Verification items for this drawing (mm, ordinates from the low corner). Coordinates: 2 decimals unless noted, no trailing zeros. Order: outer loops, then holes, each group sorted by start corner. A loop starts at its lowest first (then second) coordinate and runs counter-clockwise, first axis right, second up. Notation, with made-up numbers: (69, 60.25) -> (108, 60.25) arc R6 ccw to (108, 64.25) -> close; hole circle Ø6 at (-7.75, -8.75). An arc over 180 degrees is marked (long way). Answer as CSV lines item,"result". Start each with the question number.
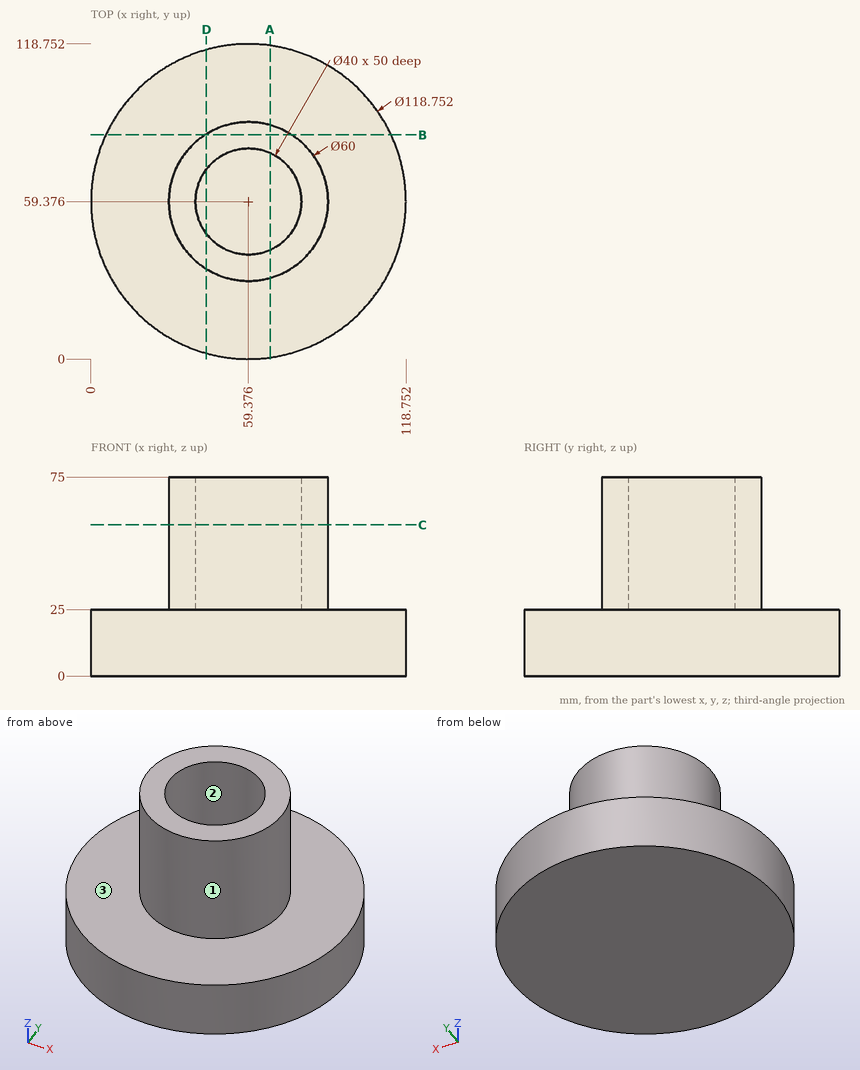
Q1. Sectioned sample at D-D, the plane x = 43.5. Record the cut outline in (y, z), then the cut area to 3 significant figures.
Q2. Go/stop test with flat-tipped pins: pin 1 Ø10 at (x, z) = (65.5, 16) entering from -Y; pin 2 Ø10 at (y, z) = (96.5, 20) entering from +X; pin 3 Ø10 at (x, z) = (85.5, 54.5) entering from -Y (1 decimal). Record where each tip stops, or that it passes through.
Q3. Sectioned sample at B-B, the plane y = 84.5. Record the cut outline in (x, z).
Q4. Sectioned sample at C-C, the plane z = 57. Record the cut outline in (x, y).
Q5. Sectioned sample at A-A, the plane x = 67.5. Record the cut outline in (y, z) (1 decimal), then the cut area to 3 significant figures.
Q6. Thickness scan on L1, parallel to Z at x = 92.5, y = 91; L2, parallel to Y at x = 45, z = 43 (1 decimal); L3, parallel to Y at x = 65, z = 32.5. Record the ranges inside material, lowest first.
Q7. Release check for a two-part mould opening along X. For the marked faces 1, 2 and 3 record: released by +X, released by -X, zero draft, split by the parting line, or undercut.
Geometry results:
1,outline,"(2.16, 0) -> (116.59, 0) -> (116.59, 25) -> (84.83, 25) -> (84.83, 75) -> (71.54, 75) -> (71.54, 25) -> (47.21, 25) -> (47.21, 75) -> (33.92, 75) -> (33.92, 25) -> (2.16, 25) -> close"
1,area,"4,190 mm^2"
2,pin 1,"stops at y = 0.01"
2,pin 2,"stops at x = 109.31"
2,pin 3,"stops at y = 38.1"
3,outline,"(5.58, 0) -> (113.17, 0) -> (113.17, 25) -> (75.77, 25) -> (75.77, 75) -> (42.98, 75) -> (42.98, 25) -> (5.58, 25) -> close"
4,outline,"circle Ø60 at (59.38, 59.38); hole circle Ø40 at (59.38, 59.38)"
5,outline,"(0.6, 0) -> (118.2, 0) -> (118.2, 25) -> (88.3, 25) -> (88.3, 75) -> (77.7, 75) -> (77.7, 25) -> (41.1, 25) -> (41.1, 75) -> (30.5, 75) -> (30.5, 25) -> (0.6, 25) -> close"
5,area,"4,000 mm^2"
6,L1,"z = 0 to 25"
6,L2,"y = 33 to 45.5, 73.3 to 85.7"
6,L3,"y = 29.91 to 40.18, 78.57 to 88.84"
7,face 1,"split by the parting line"
7,face 2,"undercut"
7,face 3,"zero draft"
